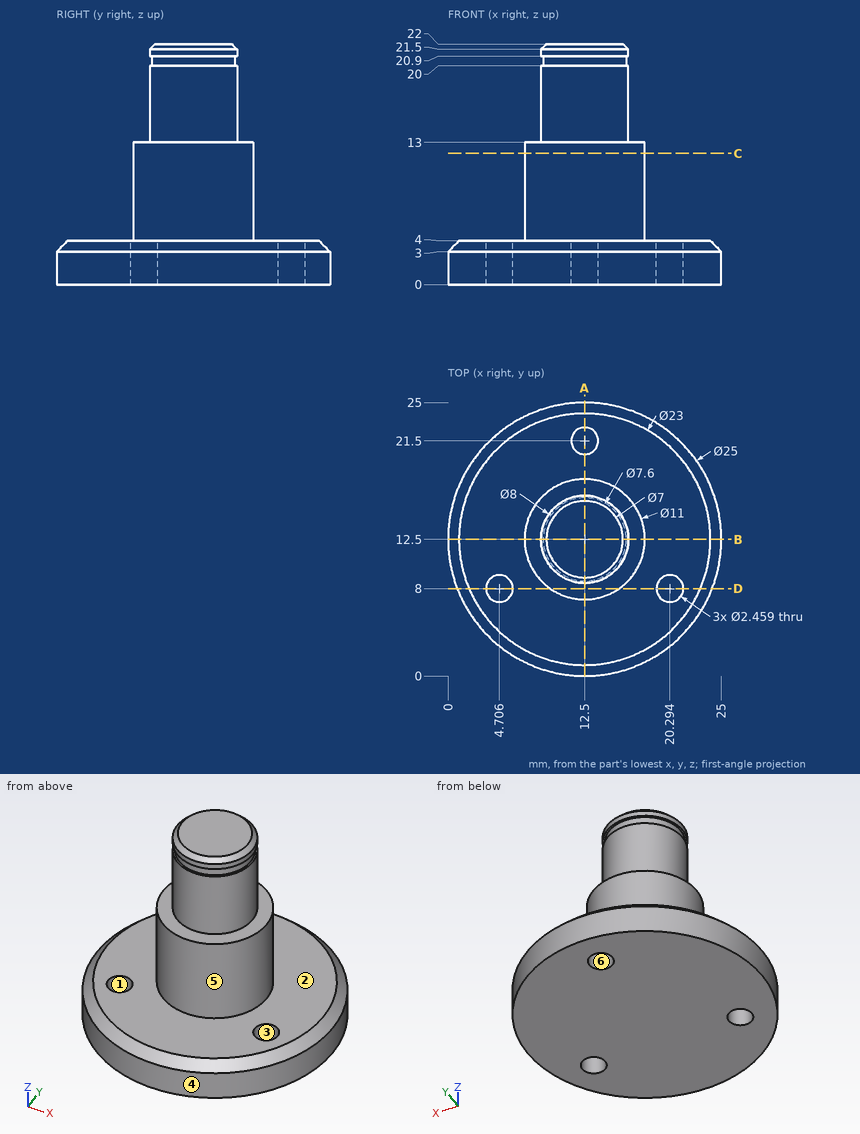
Design review of the part shown in the three views and the two pictorial views. Dimensions are in mm from the part's minimum x, y and z. A direction names the side the tool comes from. Coordinates: 2 decimals unless noted, no trailing zeros. Write each loop counter-clockwise with the first axis right and the second up, starting at its lowest first coordinate (ties: lowest second). Pieces come first, ordered by that corner, then holes. Notation, with made-up numbers: (60.5, 41.5) -> (65.5, 41.5) arc R25 cw to (65.5, 73.5) -> close; hole circle Ø9 at (47.5, -3). An arc over 180 degrees is marked (long way). Answer in a Markdown table with one row per item.
1. Draft analysis for pull direction X (two halves, no side actions). For the marked faces 1, 2, 3 and 4, state which applies: +X half, -X half, draft (parallel to the pull), parting line (faces both ways), or undercut.
Answers below:
| item | result |
|---|---|
| face 1 | undercut |
| face 2 | draft |
| face 3 | undercut |
| face 4 | parting line |
2. We need section A-A, the plane x = 12.5. State the section outline as (y, z) points.
Answers below:
| item | result |
|---|---|
| outline | (0, 0) -> (20.27, 0) -> (20.27, 4) -> (18, 4) -> (18, 13) -> (16.5, 13) -> (16.5, 20) -> (16.3, 20) -> (16.3, 20.9) -> (16.5, 20.9) -> (16.5, 21.5) -> (16, 22) -> (9, 22) -> (8.5, 21.5) -> (8.5, 20.9) -> (8.7, 20.9) -> (8.7, 20) -> (8.5, 20) -> (8.5, 13) -> (7, 13) -> (7, 4) -> (1, 4) -> (0, 3) -> close; (22.73, 0) -> (25, 0) -> (25, 3) -> (24, 4) -> (22.73, 4) -> close |
3. We need section C-C, the plane z = 12. State the section outline as (x, y) points.
Answers below:
| item | result |
|---|---|
| outline | circle Ø11 at (12.5, 12.5) |
4. Clearance check with flat-ended pins moving along their axes: pin 1 Ø1 at (x, y) = (14.5, 5.5) entering from +Z; pin 2 Ø6 at (x, z) = (6.5, 4.5) entering from -Y. State where each tip first meets the part, or that it passes through.
Answers below:
| item | result |
|---|---|
| pin 1 | stops at z = 4 |
| pin 2 | stops at y = 0.47 |
5. For the marked faces 5 and 6, list the 3-axis set-ups (+Z, -Z, +X, -X, +Y, -Y) from which the entire face can be reached by the end or side of a thin tool; tool diameter is ignored.
Answers below:
| item | result |
|---|---|
| face 5 | +Z |
| face 6 | +Z, -Z |
6. Wall thickness on probe 1 along Y at (x, z) = (12.5, 2.1); probe 2 along X at (y, z) = (8, 1.2) (1 decimal); probe 3 along Y at (x, z) = (11, 20.25): over which ranges is each line inside the solid? List them lowest first. Write a range as [from, to].
Answers below:
| item | result |
|---|---|
| probe 1 | y = [0, 20.27], [22.73, 25] |
| probe 2 | x = [0.8, 3.5], [5.9, 19.1], [21.5, 24.2] |
| probe 3 | y = [9.01, 15.99] |
7. We need section B-B, the plane y = 12.5. State the section outline as (x, z) points, and give its area (3 significant figures).
Answers below:
| item | result |
|---|---|
| outline | (0, 0) -> (25, 0) -> (25, 3) -> (24, 4) -> (18, 4) -> (18, 13) -> (16.5, 13) -> (16.5, 20) -> (16.3, 20) -> (16.3, 20.9) -> (16.5, 20.9) -> (16.5, 21.5) -> (16, 22) -> (9, 22) -> (8.5, 21.5) -> (8.5, 20.9) -> (8.7, 20.9) -> (8.7, 20) -> (8.5, 20) -> (8.5, 13) -> (7, 13) -> (7, 4) -> (1, 4) -> (0, 3) -> close |
| area | 269 mm^2 |
8. We need section D-D, the plane y = 8. Give the number of separate pieces and of enclosed holes in the cut face, and give its area (3 significant figures).
Answers below:
| item | result |
|---|---|
| separate pieces | 3 |
| enclosed holes | 0 |
| area | 129 mm^2 |
